Work out the finished part from the listing and answer in its coordinate system (mm). Coordinates: 2 decimals unless noted, no trailing zeros. Order: outer loops, then holes, each group sorted by start corner. A loop starts at its lowest first (then second) coordinate and runs counter-clockwise, first axis right, second up.
1. A flat-ended cylindrical pin translates along its axis: pin 1 Ø2 at (x, z) = (72.5, 3) entering from +Y. Find the tip coordinate at first contact, or state that the pin passes through.
2. Find the intervals of material crossed by probe 1 along Y at (x, z) = (16.5, 0.5); probe 2 along Y at (x, z) = (12, 2.9); probe 3 along X at (y, z) = (258.5, 1.85), in increasing order.
3. The part is cut by section A-A, the plane z = 2.95. Give the vertices of the cut face in (x, y), then the cut area to 3 significant figures.
4. The part is cut by section C-C, the plane x = 74. Give the vertices of the cut face in (y, z), then the cut area to 3 significant figures.
5. The part is cut by section B-B, the plane y = 227.5. Give the vertices of the cut face in (x, z), then the cut area to 3 significant figures.
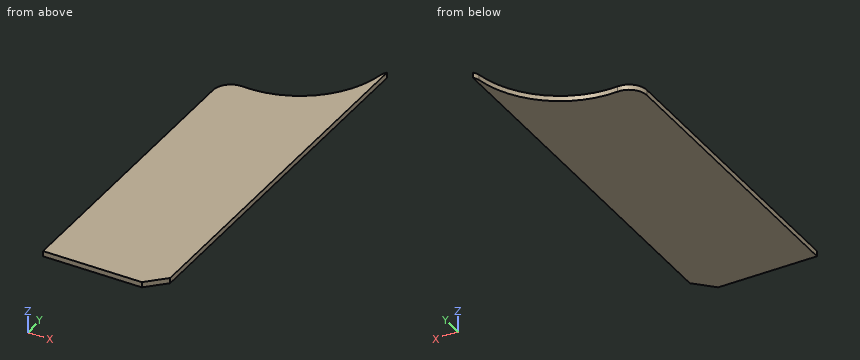
Autodesk Inventor part; units mm, degrees
ref_plane "YZ Plane" through (0, 0, 0) normal (1, 0, 0) x (0, 1, 0)
ref_plane "XZ Plane" through (0, 0, 0) normal (0, 1, 0) x (-1, 0, 0)
ref_plane "XY Plane" through (0, 0, 0) normal (0, 0, 1) x (1, 0, 0)
sketch "Sketch1" plane through (0, 0, 0) normal (0, 0, 1) x (1, 0, 0)
  line L0 (0, 0) -> (82.55, 0)
  line L1 (82.55, 0) -> (82.55, 304.8)
  line L2 (82.55, 304.8) -> (0, 304.8)
  line L3 (0, 304.8) -> (0, 0)
  dimension "d0" = 82.55
  dimension "d1" = 304.8
extrude "Extrusion1" add sketch "Sketch1" along normal blind 3.81
chamfer "Chamfer1" distance 12.7 angle 45 1 edges at (82.55, 0, 1.905)
hole "Hole1" at (17.78, 284.48, 3.81) direction (0, 0, -1) diameter 127 end through all
hole "Hole2" at (80.6545, 302.7787, 3.81) direction (0, 0, -1) diameter 48.26 end through all
fillet "Fillet1" radius 7.62 1 edges at (81.0119, 278.6513, 1.905)
fillet "Fillet2" radius 12.7 1 edges at (0, 223.52, 1.905)
properties part number "Backstopleft"
Geometry says:
1. pin 1: stops at y = 254.02
2. probe 1: y = 0 to 220.99
2. probe 2: y = 0 to 221.13
2. probe 3: x = 75.72 to 82.55
3. outline: (0, 0) - (69.85, 0) - (82.55, 12.7) - (82.55, 278.72) arc R7.62 ccw to (80.51, 274.62) arc R63.5 cw to (13.55, 221.12) arc R12.7 ccw to (0, 208.45) - close
3. area: 19,100 mm2
4. outline: (4.15, 0) - (254.96, 0) - (254.96, 3.81) - (4.15, 3.81) - close
4. area: 956 mm2
5. outline: (45.81, 0) - (82.55, 0) - (82.55, 3.81) - (45.81, 3.81) - close
5. area: 140 mm2
